For this review, take the finished solid that the model builds, in its own axes (mm). A direction names the side the tool comes from. Round coordinates to 2 decimals unless told otherwise and drop trailing zeros. Order: outer loops, then holes, each group sorted by start corner. A loop starts at its lowest first (then second) coordinate and runs counter-clockwise, first axis right, second up. Notation, with made-up numbers: (41, 22) -> (58, 22) arc R9 ccw to (58, 31) -> close; hole circle Ø7 at (67, -17.75). An arc over 180 degrees is marked (long way). Answer in a Markdown table with one row per item.
Autodesk Fusion 360 part; units mm, degrees
sketch "Body Quarter" plane through (0, 0, 0) normal (0, 0, 1) x (1, 0, 0)
  arc A0 (-45, 75) -> (-50, 70) centre (-45, 70) ccw
  line L0 (-50, 50) -> (-48, 50)
  line L1 (-48, 50) -> (-48, 46)
  line L2 (-48, 46) -> (-50, 46)
  line L3 (-50, 70) -> (-50, 50)
  line L4 (0, 0) -> (0, 75)
  line L5 (0, 0) -> (-50, 0)
  line L6 (-50, 46) -> (-50, 0)
  line L7 (-31, 75) -> (-31, 73)
  line L8 (-31, 73) -> (-35, 73)
  line L9 (-35, 73) -> (-35, 75)
  line L10 (0, 75) -> (-31, 75)
  line L11 (-35, 75) -> (-45, 75)
  dimension "d12" = 2
  dimension "d13" = 4
  dimension "d14" = 25
  dimension "d16" = 50
  dimension "d25" = 4
  dimension "d26" = 2
  dimension "d27" = 15
  dimension "d28" = 75
  dimension "d50" = 5
extrude "Extrude1" add sketch "Body Quarter" along normal blind 5
chamfer "Chamfer4" distance 4.5 distance2 2 1 edges at (-50, 23, 5) measured on face at (-50, 30.6667, 3.3333)
sketch "Sketch4" plane through (0, 0, 5) normal (0, 0, 1) x (-1, 0, 0)
  line L0 (48, -46) -> (48, 0)
  line L1 (48, 0) -> (0, 0)
  line L2 (0, 0) -> (0, -75)
  line L3 (0, -75) -> (31, -75)
  line L4 (31, -75) -> (31, -73)
  line L5 (31, -73) -> (35, -73)
  line L6 (35, -73) -> (35, -75)
  line L7 (35, -75) -> (45, -75)
  arc A0 (45, -75) -> (50, -70) centre (45, -70) ccw
  line L8 (50, -70) -> (50, -50)
  line L9 (50, -50) -> (48, -50)
  line L10 (48, -50) -> (48, -46)
  line L11 (0, 0) -> (33, 0)
  line L12 (33, 0) -> (33, -40)
  line L13 (33, -40) -> (0, -40)
  line L14 (0, -40) -> (0, 0)
  dimension "d57" = 40
  dimension "d58" = 33
extrude "Extrude4" cut sketch "Sketch4" against normal blind 3 contours L1 L2 L11 L12 L13 L14
chamfer "Chamfer5" distance 3 distance2 1.5 2 edges at (-33, 20, 2) (-16.5, 40, 2) measured on face at (-33, 13.3333, 4) measured on face at (-22, 40, 4)
sketch "Sketch5" plane through (0, 0, 5) normal (0, 0, 1) x (-1, 0, 0)
  line L0 (33, -40) -> (0, -40)
  line L1 (0, -40) -> (0, -75)
  line L2 (0, -75) -> (31, -75)
  line L3 (31, -75) -> (31, -73)
  line L4 (31, -73) -> (35, -73)
  line L5 (35, -73) -> (35, -75)
  line L6 (35, -75) -> (45, -75)
  arc A0 (45, -75) -> (50, -70) centre (45, -70) ccw
  line L7 (50, -70) -> (50, -50)
  line L8 (50, -50) -> (48, -50)
  line L9 (48, -50) -> (48, -46)
  line L10 (48, -46) -> (48, 0)
  line L11 (48, 0) -> (33, 0)
  line L12 (33, 0) -> (33, -40)
  line L13 (0, -45) -> (31, -45)
  line L14 (31, -45) -> (50, -60)
extrude "Extrude5" cut sketch "Sketch5" against normal blind 1 contours L1 L2 L3 L4 L5 L6 A0 L7 L13 L14
mirror "Mirror1" about plane through (0, 0, 0) normal (1, 0, 0) of bodies 1 merged
mirror "Mirror2" about plane through (0, 0, 0) normal (0, -1, 0) of bodies 1 merged
sketch "Mech Hole" plane through (0, 0, 5) normal (0, 0, 1) x (-1, 0, 0)
  line L0 (50, -60) -> (50, -50)
  line L1 (50, -50) -> (48, -50)
  line L2 (48, -50) -> (48, -46)
  line L3 (48, 46) -> (48, 50)
  line L4 (48, 50) -> (50, 50)
  line L5 (50, 50) -> (50, 60)
  line L6 (-50, 60) -> (-50, 50)
  line L7 (-50, 50) -> (-48, 50)
  line L8 (-48, 50) -> (-48, 46)
  line L9 (-48, -46) -> (-48, -50)
  line L10 (-48, -50) -> (-50, -50)
  line L11 (-50, -50) -> (-50, -60)
  line L12 (-11.5, -35.7841) -> (11.5, -35.7841)
  line L13 (11.5, -35.7841) -> (11.5, -12.7841)
  line L14 (11.5, -12.7841) -> (-11.5, -12.7841)
  line L15 (-11.5, -12.7841) -> (-11.5, -35.7841)
  line L16 (-11.5, -35.7841) -> (11.5, -12.7841) construction
  line L17 (11.5, -35.7841) -> (-11.5, -12.7841) construction
  line L18 (48, -46) -> (48, 46)
  line L19 (-48, 46) -> (-48, -46)
  line L20 (-50, -60) -> (-31, -45)
  line L21 (-31, -45) -> (31, -45)
  line L22 (31, -45) -> (50, -60)
  line L23 (50, 60) -> (31, 45)
  line L24 (31, 45) -> (-31, 45)
  line L25 (-31, 45) -> (-50, 60)
  line L26 (-33, -40) -> (-33, 40)
  line L27 (-33, 40) -> (33, 40)
  line L28 (33, 40) -> (33, -40)
  line L29 (33, -40) -> (-33, -40)
  point P0 (0, -24.2841)
  dimension "d39" = 23
extrude "Extrude2" cut sketch "Mech Hole" against normal through all contours L12 L13 L14 L15
mirror "Mirror3" about plane through (0, 0, 0) normal (0, 1, 0) of "Extrude2"
equation "d16 = ( 100 / 2 ) * 1 mm"
equation "d28 = ( 150 / 2 ) * 1 mm"
Q1. Take a section at D-D, the plane y = -64.5. Write out the cut boundary in (x, z), then the cut area to 3 significant figures.
Answer key:
| item | result |
|---|---|
| outline | (-50, 0) -> (50, 0) -> (50, 4) -> (-50, 4) -> close |
| area | 400 mm^2 |
Q2. To check wall thickness, follow probe 1 along Y at (x, z) = (3, 1.7); probe 2 along Z at (x, y) = (24.5, -52); probe 3 along Z at (x, y) = (0, -2). State the ranges of each line that lie inside material, in increasing order.
Answer key:
| item | result |
|---|---|
| probe 1 | y = -75 to -35.78, -12.78 to 12.78, 35.78 to 75 |
| probe 2 | z = 0 to 4 |
| probe 3 | z = 0 to 2 |
Q3. The part is to be moulded in two halves that separate along X. For faces 4 (the face through (-40.633, -52.605, 4.507)), 5 (the face through (48, 48, 2)), 6 (the face through (-48, 48, 2)), say which applies: +X half, -X half, draft (parallel to the pull), parting line (faces both ways), or undercut.
Answer key:
| item | result |
|---|---|
| face 4 | undercut |
| face 5 | +X half |
| face 6 | -X half |
Q4. Take a section at B-B, the plane x = -9.5. Give the number of separate pieces and of enclosed holes in the cut face, then the cut area to 3 significant figures.
Answer key:
| item | result |
|---|---|
| separate pieces | 3 |
| enclosed holes | 0 |
| area | 362 mm^2 |
Q5. Clearance check with flat-ended pins moving along their axes: pin 1 Ø6 at (x, y) = (-11.5, -23) entering from +Z; pin 2 Ø2 at (x, z) = (-49, 1.5) entering from -Y; pin 3 Ø1 at (x, z) = (49, 3.5) entering from +Y. State where each tip first meets the part, or that it passes through.
Answer key:
| item | result |
|---|---|
| pin 1 | stops at z = 2 |
| pin 2 | stops at y = -74 |
| pin 3 | stops at y = 73.57 |
Q6. Tool access review of faces 1 (the face through (-33, 73, 2)), 2 (the face through (40.633, 52.605, 4.507)), 3 (the face through (32, 1, 3)): name each direction out of +Z, -Z, +X, -X, +Y, -Y from which nothing blocks a thin tool from reaching the whole face with its end or side.
Answer key:
| item | result |
|---|---|
| face 1 | +Z, -Z, +Y |
| face 2 | +Z, +Y |
| face 3 | +Z |
